Can you work these out from the drawing? Everything is in mm from the part's minimum corner. A direction names the side the tool comes from. Give positions to 0.01 mm unless a question says otherwise; leave off trailing zeros. Write each loop counter-clockwise with the first axis right and the second up, starting at its lowest first coordinate (ties: lowest second). Pieces come first, ordered by that corner, then holes. Notation, with made-up numbers: (-28, -9.75) -> (-24, -9.75) arc R16 ccw to (-24, 14.25) -> close; hole circle Ø9 at (75.25, 10). An arc over 180 degrees is marked (long way). Write item = value, one per line. Start each with the question number.
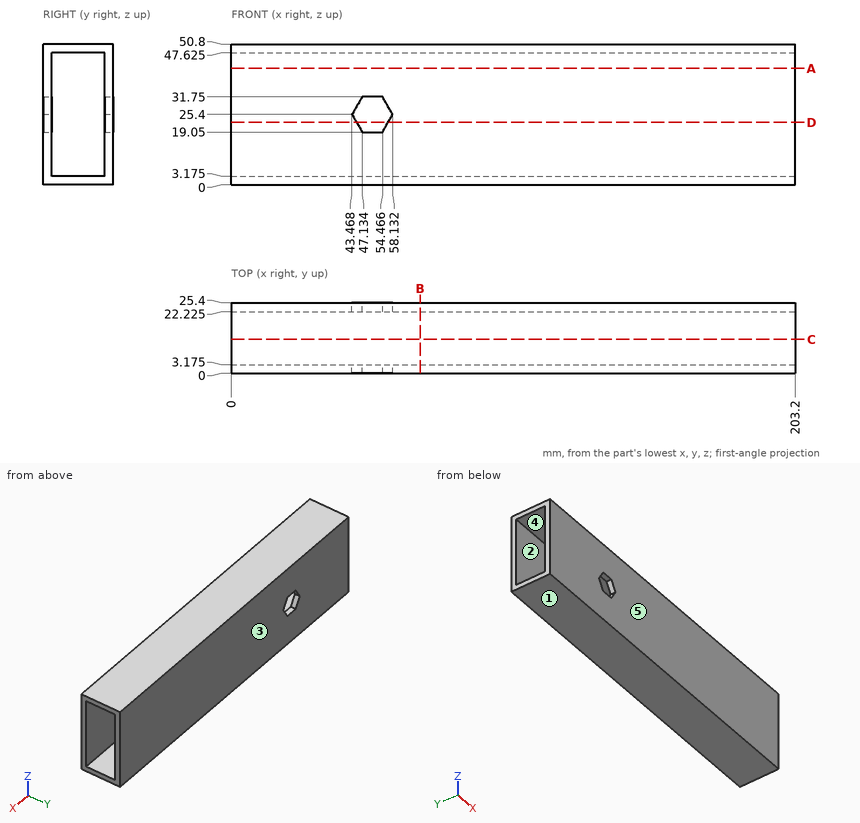
(1) If I drill on line 1 along Z through (x, y) = (80.5, 5.75) (1 decimal); line 2 along Y through (x, z) = (29, 26) (1 decimal); line 3 along Z through (x, y) = (47.5, 23.75), over which ranges is the centre line in solid material (lowest first)? Write a range as from..to.
(2) Imagine slicing it at C-C (y = 12.25). Please give me the cut outline in (x, z) (1 decimal).
(3) On a 3-axis mill with a long thin cutter (end or side, diameter ignored), from which of +Z, -Z, +X, -X, +Y, -Y can I reach the whole of each face in a straight line? I mean the marked faces 1 and 2. Say none if no direction works.
(4) Imagine slicing it at D-D (z = 22.5). Please give me the cut outline in (x, y) (1 decimal), then the cut area to 3 significant figures.
(5) Imagine slicing it at A-A (z = 42). Please give me the cut outline in (x, y) (1 decimal), then the cut area to 3 significant figures.
(6) Imagine slicing it at B-B (x = 68). Please give me the cut outline in (y, z) (1 decimal).
(7) We'd pull the mould along Y, two halves only. Please class the marked faces 3, 4 and 5: released by +Y, released by -Y, zero draft, split by the parting line, or undercut.
Answers below:
q1.line_1 = 0..3.2, 47.6..50.8
q1.line_2 = 0..3.2, 22.2..25.4
q1.line_3 = 0..19.05, 31.75..50.8
q2.outline = (0, 0) -> (203.2, 0) -> (203.2, 3.2) -> (0, 3.2) -> close; (0, 47.6) -> (203.2, 47.6) -> (203.2, 50.8) -> (0, 50.8) -> close
q3.face_1 = -Z, +X, -X, +Y, -Y
q3.face_2 = +X, -X
q4.outline = (0, 0) -> (45.1, 0) -> (45.1, 3.2) -> (0, 3.2) -> close; (0, 22.2) -> (45.1, 22.2) -> (45.1, 25.4) -> (0, 25.4) -> close; (56.5, 0) -> (203.2, 0) -> (203.2, 3.2) -> (56.5, 3.2) -> close; (56.5, 22.2) -> (203.2, 22.2) -> (203.2, 25.4) -> (56.5, 25.4) -> close
q4.area = 1,220 mm^2
q5.outline = (0, 0) -> (203.2, 0) -> (203.2, 3.2) -> (0, 3.2) -> close; (0, 22.2) -> (203.2, 22.2) -> (203.2, 25.4) -> (0, 25.4) -> close
q5.area = 1,290 mm^2
q6.outline = (0, 0) -> (25.4, 0) -> (25.4, 50.8) -> (0, 50.8) -> close; hole (3.2, 3.2) -> (22.2, 3.2) -> (22.2, 47.6) -> (3.2, 47.6) -> close
q7.face_3 = released by +Y
q7.face_4 = undercut
q7.face_5 = released by -Y
